Work out the finished part from the listing and answer in its coordinate system (mm). A direction names the side the tool comes from. Round coordinates to 2 decimals unless told otherwise and drop trailing zeros. Order: outer loops, then holes, each group sorted by start corner. A loop starts at its lowest first (then second) coordinate and runs counter-clockwise, first axis right, second up. Notation, with made-up numbers: (61, 32) - (95, 32) arc R31 cw to (95, 56) - close; hole circle Ø5 at (67, -18). An arc over 180 degrees is marked (long way). Use one line per item in the form item = value. Start each with the question number.
Q1. The part is cut by section A-A on x = -6.5. Determine the outline of the cut face in (y, z).
Q2. Find the intervals of material crossed by line 1 (Z direction, x = -4.5, y = 0.4); line 2 (X direction, y = 1.7, z = -5.5); line 3 (X direction, y = 0.25, z = -5), in increasing order. Write a range as [from, to].
Q3. The part is cut by section C-C on z = -24. Determine the outline of the cut face in (x, y).
Q4. For a pull along Z with two mould halves and no side action, classify faces 1 (the flat face through (-1.9, 1, -10)), 2 (the flat face through (-4, 0, -16)), 3 (the flat face through (-1.232, 1.014, -3.042)) as +Z half, -Z half, draft (parallel to the pull), parting line (faces both ways), or undercut.
Q5. The part is cut by section D-D on x = -1.5. Determine the outline of the cut face in (y, z), plus the area to 3 significant figures.
Q6. The part is cut by section B-B on y = 1. Determine the outline of the cut face in (x, z), plus the area to 3 significant figures.
Q7. Which of the six approach directions +Z, -Z, +X, -X, +Y, -Y give full straight-line access (tool end or side, diameter ignored) to faces 4 (the flat face through (-4, 1, -9.1)), 5 (the flat face through (-4, 2, -16))?
Autodesk Inventor part; units mm, degrees
ref_plane "YZ Plane" through (0, 0, 0) normal (1, 0, 0) x (0, 1, 0)
ref_plane "XZ Plane" through (0, 0, 0) normal (0, 1, 0) x (-1, 0, 0)
ref_plane "XY Plane" through (0, 0, 0) normal (0, 0, 1) x (1, 0, 0)
sketch "Sketch1" plane through (0, 0, 0) normal (0, 1, 0) x (-1, 0, 0)
  line L0 (0, 0) -> (7, 0)
  line L1 (7, 0) -> (7, -31.8)
  line L2 (7, -31.8) -> (0, -31.8)
  line L3 (0, -31.8) -> (0, 0)
  line L4 (7, -9.1) -> (1.9, -9.1)
  line L5 (1.9, -9.1) -> (1.9, -11.2)
  line L6 (1.9, -11.2) -> (7, -11.2)
  line L7 (7, -11.2) -> (7, -9.1)
  point P0 (7, -11.2)
  dimension "d0" = 7
  dimension "d1" = 31.8
  dimension "d2" = 2.1
  dimension "d3" = 5.1
  dimension "d4" = 9.1
extrude "Extrusion1" add sketch "Sketch1" along normal blind 2 contours L0 L1 L4 L5 L6 L2 L3
chamfer "Chamfer1" distance 2.5 distance2 6 1 edges at (0, 1, 0) measured on face at (-4.6667, 0.6667, 0)
chamfer "Chamfer2" distance 18 distance2 3 1 edges at (0, 1, -31.8) measured on face at (0, 0.6667, -14.6)
properties part number "Feather_0_aerofoil_frame_support_p2"
Found:
q1.outline = (0, -31.8) - (2, -31.8) - (2, -11.2) - (0, -11.2) - close; (0, -9.1) - (2, -9.1) - (2, 0) - (0, 0) - close
q2.line_1 = [-31.8, -11.2], [-9.1, 0]
q2.line_2 = [-7, -0.21]
q2.line_3 = [-7, -0.42]
q3.outline = (-7, 0) - (-1.7, 0) - (-1.7, 2) - (-7, 2) - close
q4.face_1 = undercut
q4.face_2 = draft
q4.face_3 = +Z half
q5.outline = (0, -22.8) - (2, -22.8) - (2, -2.4) - (0, -2.4) - close
q5.area = 40.8 mm²
q6.outline = (-7, -31.8) - (-3, -31.8) - (0, -13.8) - (0, -6) - (-2.5, 0) - (-7, 0) - (-7, -9.1) - (-1.9, -9.1) - (-1.9, -11.2) - (-7, -11.2) - close
q6.area = 177 mm²
q7.face_4 = -X, +Y, -Y
q7.face_5 = +Z, -Z, +X, -X, +Y
